Answer from the drawing. Dimensions are ordinates in mm from the lowest x, y and z of the part. A direction names the side the tool comes from. Give positions to 0.01 mm unless a question says otherwise; leave off trailing zeros. Order: outer loops, then holes, each group sorted by start corner. A loop starts at its lowest first (then second) coordinate and runs counter-clockwise, first axis right, second up.
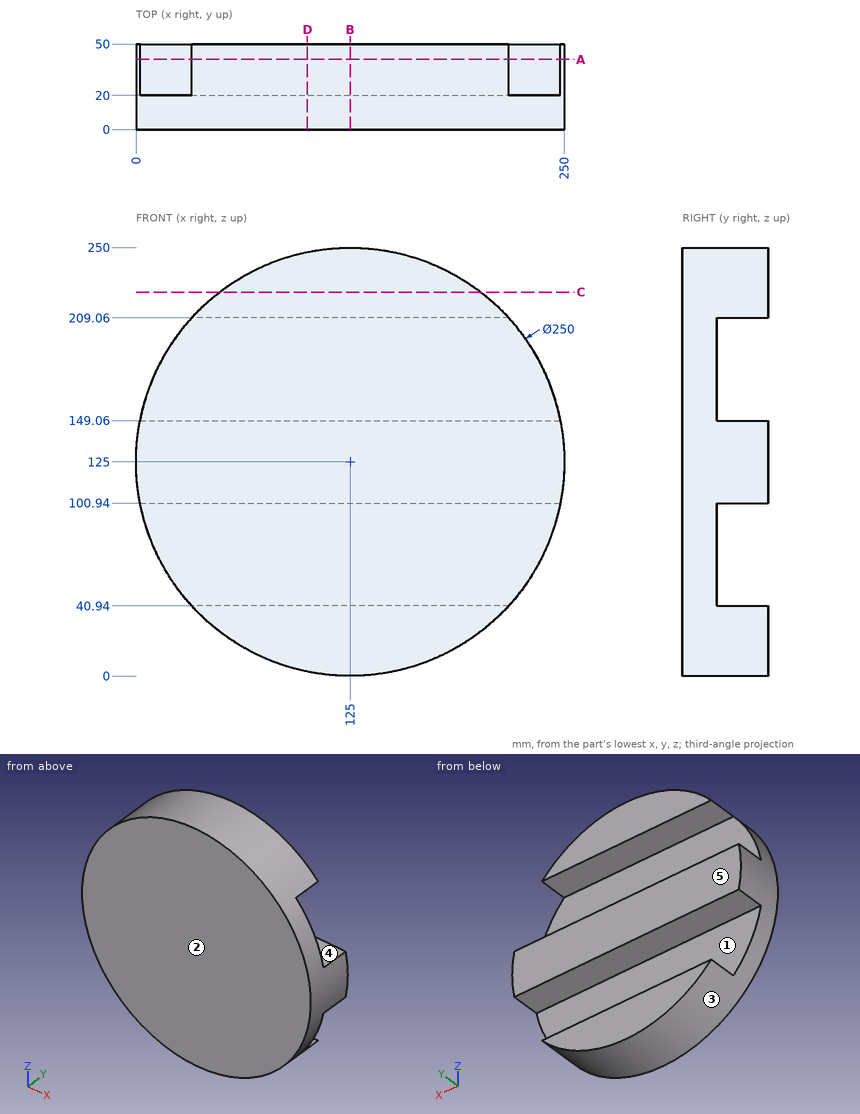
1) The part is cut by section D-D on x = 100. Determine the outline of the cut face in (y, z).
Final values:
outline: (0, 2.53) - (50, 2.53) - (50, 40.94) - (20, 40.94) - (20, 100.94) - (50, 100.94) - (50, 149.06) - (20, 149.06) - (20, 209.06) - (50, 209.06) - (50, 247.47) - (0, 247.47) - close
2) The part is cut by section C-C on z = 224. Determine the outline of the cut face in (x, y).
Final values:
outline: (48.68, 0) - (201.32, 0) - (201.32, 50) - (48.68, 50) - close
3) The part is cut by section B-B on x = 125. Determine the outline of the cut face in (y, z), and give its area (3 significant figures).
Final values:
outline: (0, 0) - (50, 0) - (50, 40.94) - (20, 40.94) - (20, 100.94) - (50, 100.94) - (50, 149.06) - (20, 149.06) - (20, 209.06) - (50, 209.06) - (50, 250) - (0, 250) - close
area: 8,900 mm2
4) Consider L1, parallel to Z at x = 129, y = 33; L2, parallel to Z at x = 109, y = 30; L3, parallel to Y at x = 208.5, z = 163. Determine where each line is inside the solid, lowest interval first.
Final values:
L1: z = 0.06 to 40.94, 100.94 to 149.06, 209.06 to 249.94
L2: z = 1.03 to 40.94, 100.94 to 149.06, 209.06 to 248.97
L3: y = 0 to 20
5) A tool of negligible diameter and unlimited length cuts with its end or side. For the marked faces 1 and 2, from which of +Z, -Z, +X, -X, +Y, -Y can it reach the whole face along a straight path? Write none if from no direction.
Final values:
face 1: +X, -X, +Y
face 2: +Z, -Z, +X, -X, -Y
6) For a pull along Z with two mould halves and no side action, classify the marked faces 3, 4 and 5 as released by +Z, released by -Z, zero draft, split by the parting line, or undercut.
Final values:
face 3: split by the parting line
face 4: undercut
face 5: zero draft
7) The part is cut by section A-A on y = 41. Determine the outline of the cut face in (x, z).
Final values:
outline: (2.34, 100.94) - (247.66, 100.94) arc R125 ccw to (247.66, 149.06) - (2.34, 149.06) arc R125 ccw to start; (32.49, 40.94) arc R125 ccw to (217.51, 40.94) - close; (32.49, 209.06) - (217.51, 209.06) arc R125 ccw to start
8) Given pin 1 (4 mm diameter, centred on y = 14, z = 44.5, fed in from +X); pin 2 (2 mm diameter, centred on x = 37, y = 20, fed in from +Z); pin 3 (18 mm diameter, centred on x = 150, z = 167, fed in from +Y), each flat-ended and moving along its own axis, determine where each tip first touches the part or whether it passes through.
Final values:
pin 1: stops at x = 222.28
pin 2: stops at z = 214.76
pin 3: stops at y = 20
